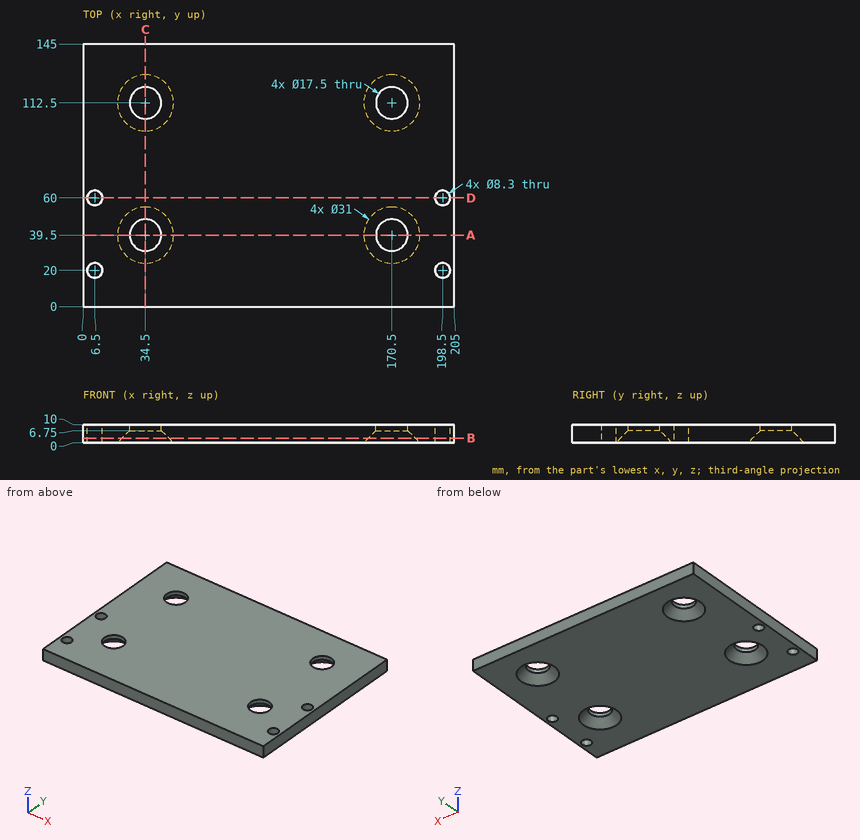
Can you work these out from the drawing? Everything is in mm from the part's minimum corner. Coordinates: 2 decimals unless noted, no trailing zeros. Loops run counter-clockwise (first coordinate to the right, second up) from the corner with the lowest first, then second, coordinate; pieces in that order, holes last.
1) For pin 1 (23 mm diameter, centred on x = 170.5, y = 112.5, fed in from -Z); pin 2 (14 mm diameter, centred on x = 34.5, y = 112.5, fed in from -Z); pin 3 (3 mm diameter, centred on x = 40, y = 107, fed in from -Z), each with a flat end and sliding along its axis, tell me the tip position at first contact or that it passes through.
2) I need wall thicknesses on probe 1 along X at (y, z) = (20, 2.75); probe 2 along X at (y, z) = (39.5, 9.2); probe 3 along Y at (x, z) = (6.5, 3). Which ranges of each line are inside material? Lowest first, please.
3) Imagine slicing it at B-B on z = 2.5. State how many separate pieces and enclosed holes the cut face has, plus the area to 3 significant figures.
4) Imagine slicing it at D-D on y = 60. List the corners of the cut face in (x, z) for me, plus the area to 3 significant figures.
5) Imagine slicing it at A-A on y = 39.5. List the corners of the cut face in (x, z) for me, plus the area to 3 significant figures.
6) Imagine slicing it at C-C on x = 34.5. List the corners of the cut face in (y, z) for me, plus the area to 3 significant figures.
Completed:
1. pin 1: stops at z = 4
1. pin 2: passes through
1. pin 3: stops at z = 6.22
2. probe 1: x = 0 to 2.35, 10.65 to 194.35, 202.65 to 205
2. probe 2: x = 0 to 25.75, 43.25 to 161.75, 179.25 to 205
2. probe 3: y = 0 to 15.85, 24.15 to 55.85, 64.15 to 145
3. separate pieces: 1
3. enclosed holes: 8
3. area: 27,400 mm2
4. outline: (0, 0) - (2.35, 0) - (2.35, 10) - (0, 10) - close; (10.65, 0) - (194.35, 0) - (194.35, 10) - (10.65, 10) - close; (202.65, 0) - (205, 0) - (205, 10) - (202.65, 10) - close
4. area: 1,880 mm2
5. outline: (0, 0) - (19, 0) - (25.75, 6.75) - (25.75, 10) - (0, 10) - close; (43.25, 6.75) - (50, 0) - (155, 0) - (161.75, 6.75) - (161.75, 10) - (43.25, 10) - close; (179.25, 6.75) - (186, 0) - (205, 0) - (205, 10) - (179.25, 10) - close
5. area: 1,610 mm2
6. outline: (0, 0) - (24, 0) - (30.75, 6.75) - (30.75, 10) - (0, 10) - close; (48.25, 6.75) - (55, 0) - (97, 0) - (103.75, 6.75) - (103.75, 10) - (48.25, 10) - close; (121.25, 6.75) - (128, 0) - (145, 0) - (145, 10) - (121.25, 10) - close
6. area: 1,010 mm2
